Design review of the part shown in the three views and the two pictorial views. Dimensions are in mm from the part's minimum x, y and z. Give positions to 0.01 mm unless a question says otherwise; leave off trailing zeros. Order: outer loops, then holes, each group sorted by start corner. A loop starts at its lowest first (then second) coordinate and runs counter-clockwise, first axis right, second up.
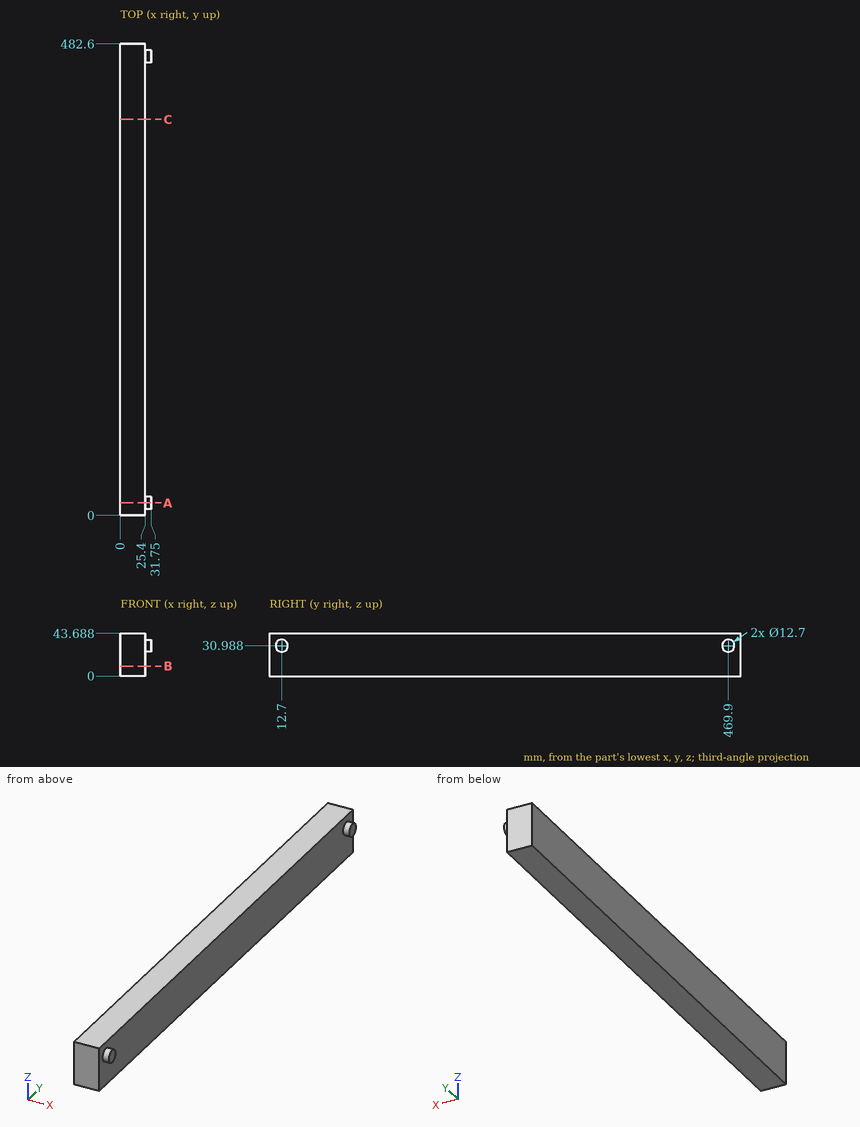
1) We need section C-C on y = 405.5. Give the boundary of the cut face in (x, z).
Answer sheet:
outline: (0, 0) - (25.4, 0) - (25.4, 43.69) - (0, 43.69) - close
2) Clearance check with a flat-ended pin moving along its axis: pin 1 (22 mm diameter, centred on y = 177.5, z = 26, fed in from +X). State where the tip first meets the part, or that it passes through.
Answer sheet:
pin 1: stops at x = 25.4
3) We need section A-A on y = 12.7. Give the boundary of the cut face in (x, z).
Answer sheet:
outline: (0, 0) - (25.4, 0) - (25.4, 24.64) - (31.75, 24.64) - (31.75, 37.34) - (25.4, 37.34) - (25.4, 43.69) - (0, 43.69) - close
4) We need section B-B on z = 10. Give the boundary of the cut face in (x, y).
Answer sheet:
outline: (0, 0) - (25.4, 0) - (25.4, 482.6) - (0, 482.6) - close
5) To check wall thickness, follow line 1 (X direction, y = 361, z = 22). State the ranges of the line that lie inside material, in increasing order.
Answer sheet:
line 1: x = 0 to 25.4
